Geometry: see drawing. Coordinates: mm, zero at the bounding-box minimum. A direction names the side the tool comes from. Coordinates: 2 decimals unless noted, no trailing zeros. Order: outer loops, then holes, each group sorted by start corner. A loop starts at its lowest first (then second) coordinate and runs counter-clockwise, first axis right, second up.
Item 1: Ray query, line 1 (Z direction, x = 1.5, y = 9.75) (1 decimal); line 2 (Z direction, x = 4.25, y = 9.5); line 3 (Y direction, x = 7.75, z = 31). Return the intervals inside material, ascending.
Item 2: Section B-B on x = 5.5. Return the cut outline in (y, z) (1 decimal).
Item 3: Section A-A on y = 6.5. Return the cut outline in (x, z) (1 decimal), then the cut area to 3 significant figures.
Item 4: Contact query for flat-ended pins moving along their axis: P1, Ø2, axis at x = 8, y = 9.5, coming from the -Z side; P2, Ø3, axis at x = 4, z = 13.5, coming from the +Y side; P3, Ø1.5, axis at y = 12.5, z = 47.5, coming from the -X side (1 decimal); P4, Ø1.5, axis at x = 2, y = 9, coming from the +Z side. Output: stop coordinate, or through.
Item 5: Reachability of the marked faces 1, 2 and 3 from +Z, -Z, +X, -X, +Y, -Y: full face, straight path, thin tool, end or side. Return the list, or none.
Item 6: Section D-D on x = 2.25. Return the cut outline in (y, z) (1 decimal).
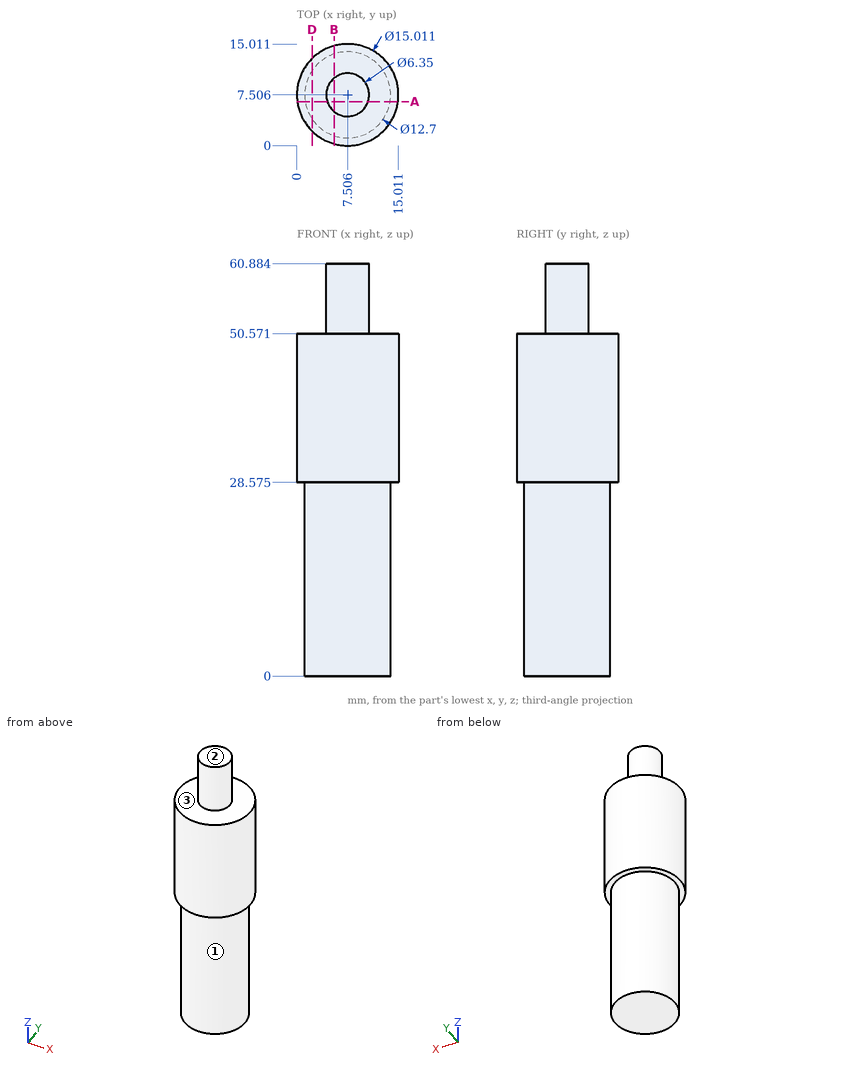
Answer list:
1. line 1: z = 28.6 to 50.6
1. line 2: z = 0 to 50.57
1. line 3: y = 0 to 15.01
2. outline: (0.3, 28.6) - (1.5, 28.6) - (1.5, 0) - (13.5, 0) - (13.5, 28.6) - (14.7, 28.6) - (14.7, 50.6) - (10, 50.6) - (10, 60.9) - (5, 60.9) - (5, 50.6) - (0.3, 50.6) - close
3. outline: (0.1, 28.6) - (1.2, 28.6) - (1.2, 0) - (13.8, 0) - (13.8, 28.6) - (14.9, 28.6) - (14.9, 50.6) - (10.5, 50.6) - (10.5, 60.9) - (4.5, 60.9) - (4.5, 50.6) - (0.1, 50.6) - close
3. area: 748 mm2
4. P1: stops at z = 0
4. P2: stops at y = 13.53
4. P3: stops at x = 1.3
4. P4: stops at z = 50.57
5. face 1: -Z
5. face 2: +Z, +X, -X, +Y, -Y
5. face 3: +Z
6. outline: (2.1, 28.6) - (3.9, 28.6) - (3.9, 0) - (11.1, 0) - (11.1, 28.6) - (12.9, 28.6) - (12.9, 50.6) - (2.1, 50.6) - close
